For this review, take the finished solid that the model builds, in its own axes (mm). A direction names the side the tool comes from. Round coordinates to 2 decimals unless told otherwise and drop trailing zeros. Order: outer loops, then holes, each group sorted by start corner. A loop starts at its lowest first (then second) coordinate and runs counter-clockwise, first axis right, second up. Notation, with made-up numbers: (87.5, 64) -> (95.5, 64) arc R22 cw to (95.5, 90) -> close; hole circle Ø11 at (36, -15). An arc over 180 degrees is marked (long way). Use a Markdown table: item, result. Add a question column.
1) Consider section D-D (y = 3). State the section outline as (x, z) points.
2) Consider section A-A (z = 0). State the section outline as (x, y) points.
3) Consider section B-B (y = 28.75). State the section outline as (x, z) points, plus the area to 3 significant figures.
4) Draft analysis for pull direction Z (two halves, no side actions). For faces 1 (the face through (-4, 35, 4)), 2 (the face through (13.9, -26.2, -8.8)), 3 (the face through (9, -30.2, -8.9)), state which applies: pulls with the +Z half, pulls with the -Z half, needs draft (parallel to the pull), parting line crosses it, or undercut.
5) Machinability: for faces 4 (the face through (12, -10, -13.157)), 5 (the face through (-9, -8, -9)), 6 (the face through (1, 0, -12)), which of the approach directions +Z, -Z, +X, -X, +Y, -Y give a long, thin tool a straight path to every point of the face, cutting with its end or side? Answer none if there is none.
6) Clearance check with flat-ended pins moving along their axes: P1, Ø5.5, axis at y = -9.58, z = -10.23, coming from the +X side; P2, Ø5.5, axis at y = 9.58, z = -10.23, coming from the -X side; P3, Ø3, axis at x = 9, y = -19.5, coming from the -Z side. State where each tip first meets the part, or that it passes through.
7) Consider section C-C (x = -16.5). State the section outline as (y, z) points.
8) Wall thickness on line 1 along Y through (x, z) = (-11.5, -12); line 2 along X through (y, z) = (24, -8); line 3 along Z through (x, y) = (-7.5, 8): over which ranges is each line inside the solid? List them lowest first. Write a range as [from, to].
```python
from build123d import *

# Parameters (mm, degrees)
SKETCH1_R           = 20
SKETCH1_R_2         = 4.25
BOSS_EXTRUDE1_DEPTH = 35
SKETCH2_W           = 2
SKETCH2_H           = 25
CUT_EXTRUDE1_DEPTH  = 35
SKETCH4_R           = 1.75
CUT_EXTRUDE2_DEPTH  = 30
CUT_EXTRUDE3_DEPTH  = 11
SKETCH6_R           = 3
CUT_EXTRUDE4_DEPTH  = 11


with BuildPart() as part:
    # Sketch1 → Boss-Extrude1 (new, symmetric)
    with BuildSketch(Plane(origin=(0, 0, 0), x_dir=(1, 0, 0), z_dir=(0, 1, 0))):
        with Locations(Location((0, 0, 0), (0, 0, 270))):
            Circle(SKETCH1_R)
        with Locations(Location((0, 0, 0), (0, 0, 270))):
            Circle(SKETCH1_R_2, mode=Mode.SUBTRACT)
    extrude(amount=BOSS_EXTRUDE1_DEPTH, both=True)

    # Sketch2 → Cut-Extrude1 (cut, symmetric)
    with BuildSketch(Plane(origin=(0, 0, 0), x_dir=(1, 0, 0), z_dir=(0, 1, 0))):
        with Locations((0, 12.5)):
            Rectangle(SKETCH2_W, SKETCH2_H)
    extrude(amount=CUT_EXTRUDE1_DEPTH, both=True, mode=Mode.SUBTRACT)

    # Sketch4 → Cut-Extrude2 (cut)
    with BuildSketch(Plane(origin=(20, 0, 0), x_dir=(0, 0, -1), z_dir=(1, 0, 0))):
        with Locations((10.231687805, 28.75)):
            Circle(SKETCH4_R)
        with Locations((10.231687805, 9.583333333)):
            Circle(SKETCH4_R)
        with Locations((10.231687805, -9.583333333)):
            Circle(SKETCH4_R)
        with Locations((10.231687805, -28.75)):
            Circle(SKETCH4_R)
    extrude(amount=-CUT_EXTRUDE2_DEPTH, mode=Mode.SUBTRACT)

    # Sketch5 → Cut-Extrude3 (cut)
    with BuildSketch(Plane(origin=(20, 0, 0), x_dir=(0, 0, -1), z_dir=(1, 0, 0))):
        Polygon((10.231687805, 32.127499075), (7.306687805, 30.438749537), (7.306687805, 27.061250463), (10.231687805, 25.372500925), (13.156687805, 27.061250463), (13.156687805, 30.438749537), align=None)
        Polygon((10.231687805, 6.205834259), (13.156687805, 7.894583796), (13.156687805, 11.272082871), (10.231687805, 12.960832408), (7.306687805, 11.272082871), (7.306687805, 7.894583796), align=None)
        Polygon((10.231687805, -12.960832408), (13.156687805, -11.272082871), (13.156687805, -7.894583796), (10.231687805, -6.205834259), (7.306687805, -7.894583796), (7.306687805, -11.272082871), align=None)
        Polygon((10.231687805, -32.127499075), (13.156687805, -30.438749537), (13.156687805, -27.061250463), (10.231687805, -25.372500925), (7.306687805, -27.061250463), (7.306687805, -30.438749537), align=None)
    extrude(amount=-CUT_EXTRUDE3_DEPTH, mode=Mode.SUBTRACT)

    # Sketch6 → Cut-Extrude4 (cut)
    with BuildSketch(Plane(origin=(-20, 0, 0), x_dir=(0, 0, -1), z_dir=(1, 0, 0))):
        with Locations(Location((10.231687805, 28.75, 0), (0, 0, 180))):
            Circle(SKETCH6_R)
        with Locations(Location((10.231687805, 9.583333333, 0), (0, 0, 180))):
            Circle(SKETCH6_R)
        with Locations(Location((10.231687805, -9.583333333, 0), (0, 0, 180))):
            Circle(SKETCH6_R)
        with Locations(Location((10.231687805, -28.75, 0), (0, 0, 180))):
            Circle(SKETCH6_R)
    extrude(amount=CUT_EXTRUDE4_DEPTH, mode=Mode.SUBTRACT)


solid = part.part
```
Results list:
| question | item | result |
|---|---|---|
| 1 | outline | (-1, -19.97) -> (-1, -4.13) arc R4.25 cw (long way) to (1, -4.13) -> (1, -19.97) arc R20 ccw (long way) to start |
| 2 | outline | (-20, -35) -> (-4.25, -35) -> (-4.25, 35) -> (-20, 35) -> close; (4.25, -35) -> (20, -35) -> (20, 35) -> (4.25, 35) -> close |
| 3 | outline | (-18.65, -7.23) -> (-9, -7.23) -> (-9, -8.48) -> (-1, -8.48) -> (-1, -4.13) arc R4.25 cw (long way) to (1, -4.13) -> (1, -8.48) -> (9, -8.48) -> (9, -7.31) -> (18.62, -7.31) arc R20 ccw (long way) to start; (-15, -13.23) arc R20 ccw to (-1, -19.97) -> (-1, -11.98) -> (-9, -11.98) -> (-9, -13.23) -> close; (1, -19.97) arc R20 ccw to (15.06, -13.16) -> (9, -13.16) -> (9, -11.98) -> (1, -11.98) -> close |
| 3 | area | 1,020 mm2 |
| 4 | face 1 | needs draft |
| 4 | face 2 | undercut |
| 4 | face 3 | undercut |
| 5 | face 4 | +X |
| 5 | face 5 | -X |
| 5 | face 6 | -Z, +Y, -Y |
| 6 | P1 | x = 9 |
| 6 | P2 | x = -9 |
| 6 | P3 | z = -18.54 |
| 7 | outline | (-35, -11.3) -> (-31.55, -11.3) arc R3 cw (long way) to (-25.95, -11.3) -> (-12.39, -11.3) arc R3 cw (long way) to (-6.78, -11.3) -> (6.78, -11.3) arc R3 cw (long way) to (12.39, -11.3) -> (25.95, -11.3) arc R3 cw (long way) to (31.55, -11.3) -> (35, -11.3) -> (35, 11.3) -> (-35, 11.3) -> close |
| 8 | line 1 | [-35, -31.17], [-26.33, -12.01], [-7.16, 7.16], [12.01, 26.33], [31.17, 35] |
| 8 | line 2 | [-18.33, -1], [1, 18.33] |
| 8 | line 3 | [-18.54, -10.98], [-9.49, 18.54] |
